Here's how the part is built. I have some questions about the finished solid (model axes, mm). Face numbers are marked on the shaded views. A direction names the side the tool comes from. Give positions to 0.01 mm unless a question says otherwise; leave off trailing zeros. Order: outer loops, then holes, each group sorted by start corner. A loop starts at its lowest first (then second) coordinate and runs counter-clockwise, first axis right, second up.
Autodesk Inventor part; units mm, degrees
ref_plane "YZ Plane" through (0, 0, 0) normal (1, 0, 0) x (0, 1, 0)
ref_plane "XZ Plane" through (0, 0, 0) normal (0, 1, 0) x (-1, 0, 0)
ref_plane "XY Plane" through (0, 0, 0) normal (0, 0, 1) x (1, 0, 0)
sketch "Sketch1" plane through (0, 0, 0) normal (0, 0, 1) x (1, 0, 0)
  line L0 (-12.1708, 16.0073) -> (13.2292, 16.0073)
  line L1 (13.2292, 16.0073) -> (13.2292, -34.7927)
  line L2 (13.2292, -34.7927) -> (-12.1708, -34.7927)
  line L3 (-12.1708, -34.7927) -> (-12.1708, 16.0073)
  line L4 (11.9592, 14.7373) -> (-10.9008, 14.7373)
  line L5 (-10.9008, 14.7373) -> (-10.9008, -33.5227)
  line L6 (-10.9008, -33.5227) -> (11.9592, -33.5227)
  line L7 (11.9592, -33.5227) -> (11.9592, 14.7373)
  point P0 (0, 0)
  dimension "d0" = 25.4
  dimension "d1" = 50.8
  dimension "d2" = 1.27
extrude "Extrusion1" add sketch "Sketch1" along normal blind 101.6
sketch "Sketch2" plane through (-12.1708, 16.0073, 0) normal (0, 1, 0) x (1, 0, 0)
  circle A0 centre (12.7, -12.7) radius 1.7272
  line L0 (25.4, 0) -> (0, 0)
  line L1 (0, 0) -> (0, -101.6)
  point P0 (12.1708, 0)
  dimension "d5" = 3.4544
  dimension "d6" = 12.7
  dimension "d7" = 12.7
extrude "Extrusion2" cut sketch "Sketch2" against normal through all
pattern_linear "Rectangular Pattern1" count 10 spacing 25.4 along (0, 0, 1) of "Extrusion2"
equation "\"d3\" = d13"
equation "\"d10\" = d14"
equation "\"d13\" = 101.6"
equation "\"d14\" = d13"
properties part number "wrist attatchment"
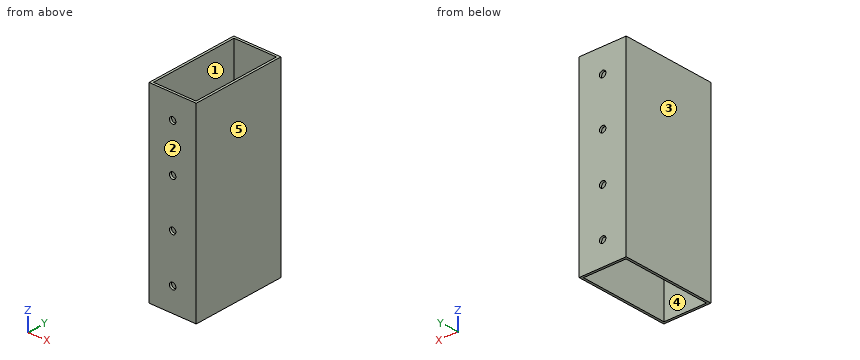
Q1. If we section it at A-A on x = 6.5: List the corners of the cut face in (y, z) for me.
Filled sheet:
outline: (-34.79, 0) - (-33.52, 0) - (-33.52, 101.6) - (-34.79, 101.6) - close; (14.74, 0) - (16.01, 0) - (16.01, 101.6) - (14.74, 101.6) - close
Q2. I need wall thicknesses on L1, parallel to Y at x = -0.5, z = 67.5; L2, parallel to X at y = 10, z = 69; L3, parallel to X at y = 15.3, z = 38.1. Which ranges of each line are inside material? Lowest first, please.
Filled sheet:
L1: y = -34.79 to -33.52, 14.74 to 16.01
L2: x = -12.17 to -10.9, 11.96 to 13.23
L3: x = -12.17 to -1.2, 2.26 to 13.23
Q3. If we section it at D-D on z = 63.5: List the corners of the cut face in (x, y) for me.
Filled sheet:
outline: (-12.17, -34.79) - (-1.2, -34.79) - (-1.2, -33.52) - (-10.9, -33.52) - (-10.9, 14.74) - (-1.2, 14.74) - (-1.2, 16.01) - (-12.17, 16.01) - close; (2.26, -34.79) - (13.23, -34.79) - (13.23, 16.01) - (2.26, 16.01) - (2.26, 14.74) - (11.96, 14.74) - (11.96, -33.52) - (2.26, -33.52) - close
Q4. For the marked faces 4 and 5, which set-ups out of +Z, -Z, +X, -X, +Y, -Y let a thin tool reach every point of the face, with its end or its side?
Filled sheet:
face 4: +Z, -Z
face 5: +Z, -Z, +X, +Y, -Y
Q5. I'm going to push a flat-ended pin straight in: P1, Ø3, axis at x = 0.53, z = 12.7, coming from the +Y side. Where does the tip first touch, or does it pass through?
Filled sheet:
P1: passes through
Q6. If we section it at B-B on y = -13.5: List the corners of the cut face in (x, z) for me.
Filled sheet:
outline: (-12.17, 0) - (-10.9, 0) - (-10.9, 101.6) - (-12.17, 101.6) - close; (11.96, 0) - (13.23, 0) - (13.23, 101.6) - (11.96, 101.6) - close
Q7. If we section it at C-C on z = 50.5: List the corners of the cut face in (x, y) for me, plus the area to 3 significant figures.
Filled sheet:
outline: (-12.17, -34.79) - (13.23, -34.79) - (13.23, 16.01) - (-12.17, 16.01) - close; hole (-10.9, -33.52) - (11.96, -33.52) - (11.96, 14.74) - (-10.9, 14.74) - close
area: 187 mm2
Q8. Thinking about a two-plate mould opening in Y: for the marked faces 1, 2 and 3, which applies, released by +Y, released by -Y, zero draft, split by the parting line, or undercut?
Filled sheet:
face 1: undercut
face 2: released by -Y
face 3: zero draft
